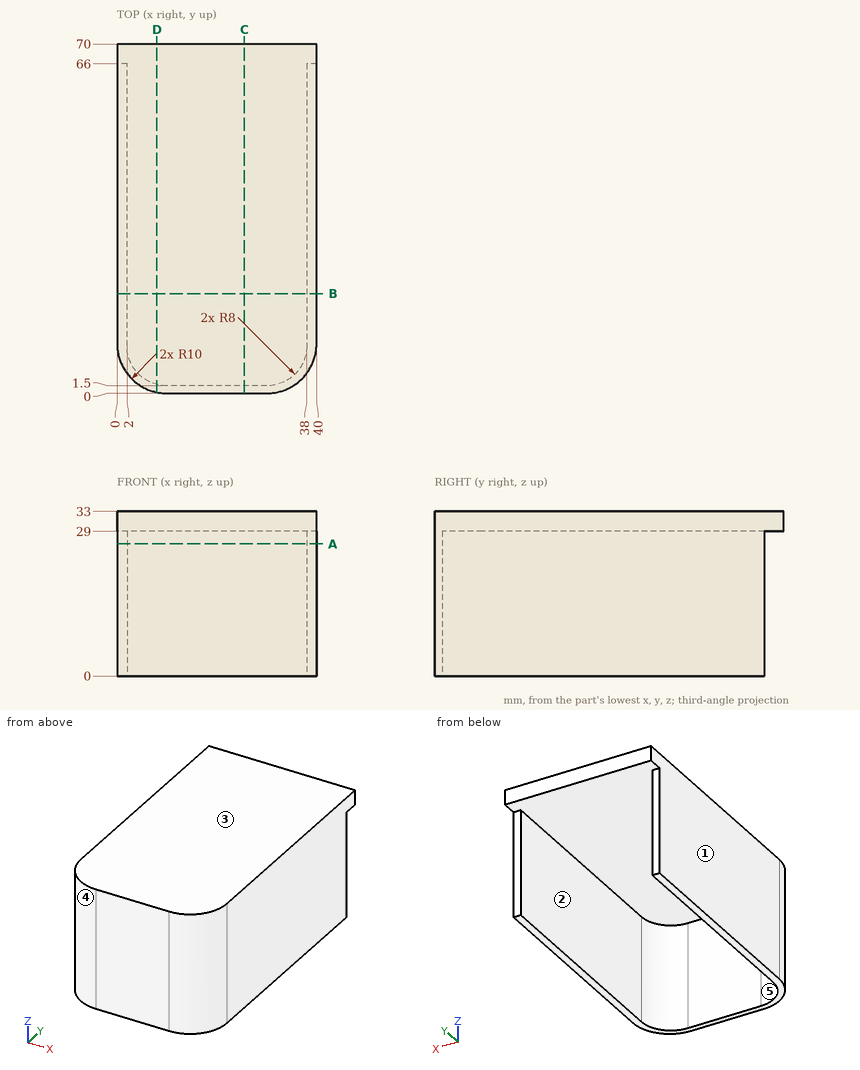
Geometry check sheet. Reference: drawing and pictorial views, mm from the part's lowest x, y, z. A direction names the side the tool comes from. Round coordinates to 2 decimals unless told otherwise and drop trailing zeros. Loops run counter-clockwise (first coordinate to the right, second up) from the corner with the lowest first, then second, coordinate; pieces in that order, holes last. Notation, with made-up numbers: M 58.25,84 L 96.25,84 A26 ccw 96.25,103 Z; hole C 3.25,-18.5 d3. An arc over 180 degrees is marked long. One line per item, written item: value.
(1) Sectioned sample at A-A, the plane z = 26.5. Record the cut outline in (x, y).
Computed values:
outline: M 0,10 A10 ccw 10,0 L 30,0 A10 ccw 40,10 L 40,66 L 38,66 L 38,9.5 A8 cw 30,1.5 L 10,1.5 A8 cw 2,9.5 L 2,66 L 0,66 Z
(2) Access from +Z, -Z, +X, -X, +Y, -Y to the whole of each face (thin tool, end or side, straight path). Record for the marked faces 4 and 5.
Computed values:
face 4: +Z, -Z, -X, -Y
face 5: -Z, +Y
(3) Thickness scan on line 1 (X direction, y = 33, z = 4); line 2 (Z direction, x = 21, y = 51); line 3 (X direction, y = 9.5, z = 29.5). Record the ranges inside material, lowest first.
Computed values:
line 1: x = 0 to 2, 38 to 40
line 2: z = 29 to 33
line 3: x = 0.01 to 39.99
(4) Sectioned sample at C-C, the plane x = 25.5. Record the cut outline in (y, z).
Computed values:
outline: M 0,0 L 1.5,0 L 1.5,29 L 70,29 L 70,33 L 0,33 Z
(5) Sectioned sample at B-B, the plane y = 20. Record the cut outline in (x, z).
Computed values:
outline: M 0,0 L 2,0 L 2,29 L 38,29 L 38,0 L 40,0 L 40,33 L 0,33 Z
(6) Release check for a two-part mould opening along X. For the marked faces 1, 2 and 3 record: +X half, -X half, draft (parallel to the pull), parting line (faces both ways), or undercut.
Computed values:
face 1: -X half
face 2: undercut
face 3: draft
(7) Depth check by flat-ended pin: pin 1 Ø12 at (x, y) = (24, 33) entering from -Z; pin 2 Ø1 at (x, z) = (39, 19.5) entering from +Y; pin 3 Ø10 at (x, z) = (16.5, 16) entering from +Y. Enter the tip coordinate at first touch or a pass-through.
Computed values:
pin 1: stops at z = 29
pin 2: stops at y = 66
pin 3: stops at y = 1.5
(8) Sectioned sample at D-D, the plane x = 8. Record the cut outline in (y, z), then the cut area to 3 significant figures.
Computed values:
outline: M 0.2,0 L 1.75,0 L 1.75,29 L 70,29 L 70,33 L 0.2,33 Z
area: 324 mm^2
